Could you check a few things on this drawing? It's one solid part, dimensions in mm from its lowest x, y, z. Give positions to 0.01 mm unless a question says otherwise; leave off trailing zeros. Loops run counter-clockwise (first coordinate to the right, second up) from the corner with the lowest first, then second, coordinate; pieces in that order, holes last. Notation, with made-up numbers: M 74,-11.75 L 82,-11.75 A13 cw 82,10.25 Z; hole C 76.25,27.25 d2. An arc over 180 degrees is marked long. One line per item, written item: value. Start each with the question number.
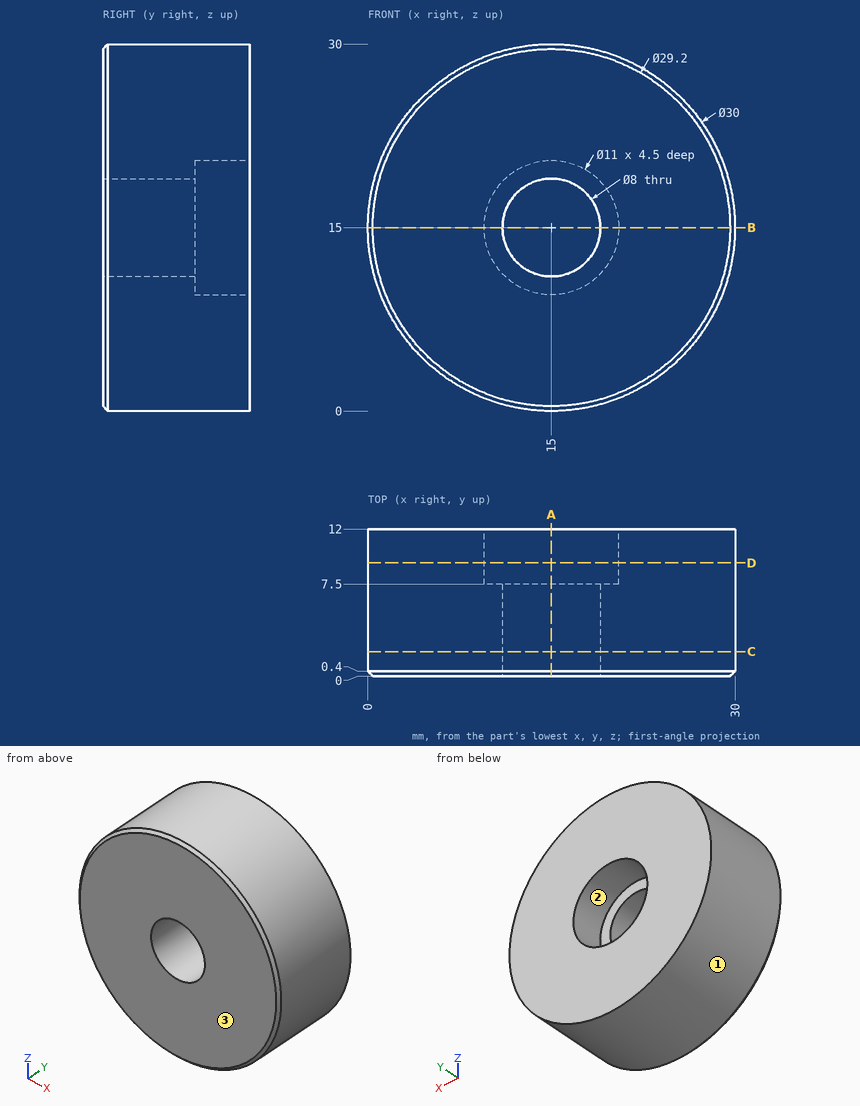
Q1. I need wall thicknesses on line 1 along X through (y, z) = (3.75, 15); line 2 along X through (y, z) = (10.55, 15); line 3 along Z through (x, y) = (10.25, 9.75). Which ranges of each line are inside material? Lowest first, please.
Q2. If we section it at A-A, the plane x = 15: Write out the boundary of the cut face in (y, z), plus the area to 3 significant figures.
Q3. If we section it at C-C, the plane y = 2: Write out the boundary of the cut face in (x, z).
Q4. For P1, Ø3, axis at x = 17, y = 5.5, coming from the -Z side; P2, Ø9, axis at x = 15, z = 14.5, coming from the +Y side; P3, Ø1.5, axis at x = 24.5, y = 3.5, coming from the +Z side, each with a flat end and sliding along its axis, tell me the tip position at first contact or that it passes through.
Q5. If we mould it in two halves opening along Z, with no side actions, what happens to the marked faces 1, 2 and 3? For each: released by +Z, released by -Z, zero draft, split by the parting line, or undercut.
Q6. If we section it at B-B, the plane z = 15: Write out the boundary of the cut face in (x, y).
Q7. If we section it at D-D, the plane y = 9.25: Write out the boundary of the cut face in (x, z).
Response:
1. line 1: 0 to 11, 19 to 30
1. line 2: 0 to 9.5, 20.5 to 30
1. line 3: 0.77 to 12.23, 17.77 to 29.23
2. outline: M 0,0.4 L 0.4,0 L 12,0 L 12,9.5 L 7.5,9.5 L 7.5,11 L 0,11 Z; M 0,19 L 7.5,19 L 7.5,20.5 L 12,20.5 L 12,30 L 0.4,30 L 0,29.6 Z
2. area: 250 mm^2
3. outline: C 15,15 d30; hole C 15,15 d8
4. P1: z = 0.01
4. P2: y = 7.5
4. P3: z = 27.18
5. face 1: split by the parting line
5. face 2: undercut
5. face 3: zero draft
6. outline: M 0,0.4 L 0.4,0 L 11,0 L 11,7.5 L 9.5,7.5 L 9.5,12 L 0,12 Z; M 19,0 L 29.6,0 L 30,0.4 L 30,12 L 20.5,12 L 20.5,7.5 L 19,7.5 Z
7. outline: C 15,15 d30; hole C 15,15 d11
